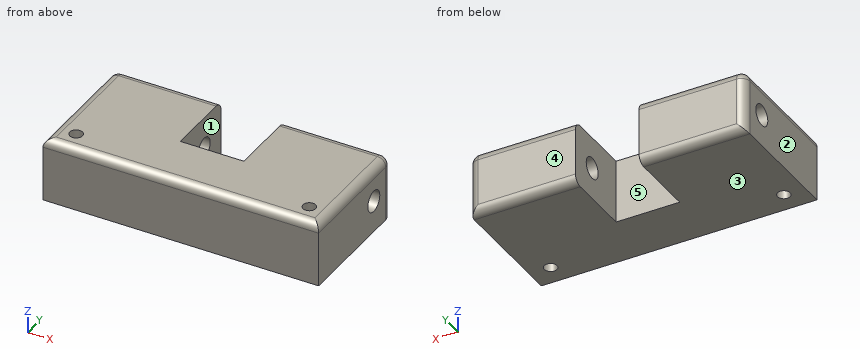
```python
from build123d import *

# Parameters (mm, degrees)
SKETCH1_W           = 65
SKETCH1_H           = 30.1
SKETCH1_R           = 1.5
BOSS_EXTRUDE1_DEPTH = 15
SKETCH2_R           = 2.5
CUT_EXTRUDE1_DEPTH  = 75
SKETCH3_W           = 15
SKETCH3_H           = 17
CUT_EXTRUDE2_DEPTH  = 75
FILLET2_R           = 2


with BuildPart() as part:
    # Sketch1 → Boss-Extrude1 (new body)
    with BuildSketch(Plane.XY):
        with Locations((10, 0.55)):
            Rectangle(SKETCH1_W, SKETCH1_H)
        with Locations((-17.5, -9.5)):
            Circle(SKETCH1_R, mode=Mode.SUBTRACT)
        with Locations((37.5, -9.5)):
            Circle(SKETCH1_R, mode=Mode.SUBTRACT)
    extrude(amount=BOSS_EXTRUDE1_DEPTH)

    # Sketch2 → Cut-Extrude1 (cut)
    with BuildSketch(Plane.ZY.offset(22.5)):
        with Locations((7.5, 8.6)):
            Circle(SKETCH2_R)
    extrude(amount=-CUT_EXTRUDE1_DEPTH, mode=Mode.SUBTRACT)

    # Sketch3 → Cut-Extrude2 (cut)
    with BuildSketch(Plane.XY.offset(15)):
        with Locations((10, 7.1)):
            Rectangle(SKETCH3_W, SKETCH3_H)
    extrude(amount=-CUT_EXTRUDE2_DEPTH, mode=Mode.SUBTRACT)

    # Fillet2
    fillet2_edges = [part.edges().sort_by_distance(p)[0] for p in [
        (42.5, 0.55, 15),
        (30, 15.6, 15),
        (-10, 15.6, 0),
        (-10, 15.6, 15),
        (-22.5, 0.55, 15),
        (30, 15.6, 0),
        (-22.5, 15.6, 7.5),
        (42.5, 15.6, 7.5),
        (10, -14.5, 15),
    ]]
    fillet(fillet2_edges, radius=FILLET2_R)


solid = part.part
```
Can you work these out from the model? Positions are in its coordinate system, mm. Face numbers are marked on the shaded views. A direction names the side the tool comes from. Give positions to 0.01 mm unless a question says otherwise; leave off trailing zeros. Loops run counter-clockwise (first coordinate to the right, second up) from the corner with the lowest first, then second, coordinate; pieces in that order, holes last. Notation, with made-up numbers: M -36,-9.5 L -10,-9.5 A22 cw -10,24.5 Z; hole C 89,-24.75 d10. An arc over 180 degrees is marked long. Use CSV: the item, a comma, the result in double quotes. Start each with the question number.
1. If I drill on L1, parallel to X at y = -0.5, z = 12; L2, parallel to Y at x = 37.5, z = 4; L3, parallel to Y at x = 31.5, z = 7.5, over which ranges is the centre line in solid material (lowest first)?
2. If we mould it in two halves opening along X, with no side actions, what happens to the marked faces 1, 2 and 3? For each: released by +X, released by -X, zero draft, split by the parting line, or undercut.
3. On a 3-axis mill with a long thin cutter (end or side, diameter ignored), from which of +Z, -Z, +X, -X, +Y, -Y can I reach the whole of each face in a straight line? I mean the marked faces 4 and 5. Say none if no direction works.
4. Imagine slicing it at A-A, the plane x = -17.5. Write out the boundary of the cut face in (y, z), plus the area to 3 significant figures.
5. Imagine slicing it at C-C, the plane z = 9. Write out the boundary of the cut face in (x, y), plus the area to 3 significant figures.
6. Imagine slicing it at B-B, the plane y = -9.5. Write out the boundary of the cut face in (x, z).
7. For P1, Ø1.8, axis at x = 37.5, y = -9.5, coming from the +Z side; P2, Ø7.5, axis at x = 6.5, z = 5, coming from the +Y side, each with a flat end and sliding along its axis, tell me the tip position at first contact or that it passes through.
8. Imagine slicing it at D-D, the plane y = 4. Write out the boundary of the cut face in (x, z).
Response values:
1,L1,"-22.5 to 2.5, 17.5 to 42.5"
1,L2,"-14.5 to -11, -8 to 15.6"
1,L3,"-14.5 to 6.1, 11.1 to 15.6"
2,face 1,"undercut"
2,face 2,"released by -X"
2,face 3,"zero draft"
3,face 4,"+Z, -Z, +X, -X, +Y"
3,face 5,"+Z, -Z, +Y"
4,outline,"M -14.5,0 L -11,0 L -11,15 L -12.5,15 A2 ccw -14.5,13 Z; M -8,0 L 13.6,0 A2 ccw 15.6,2 L 15.6,13 A2 ccw 13.6,15 L -8,15 Z; hole C 8.6,7.5 d5"
4,area,"384 mm^2"
5,outline,"M -22.5,-14.5 L 42.5,-14.5 L 42.5,6.6 L 17.5,6.6 L 17.5,-1.4 L 2.5,-1.4 L 2.5,6.6 L -22.5,6.6 Z; M -22.5,10.6 L 2.5,10.6 L 2.5,15.6 L -20.5,15.6 A2 ccw -22.5,13.6 Z; M 17.5,10.6 L 42.5,10.6 L 42.5,13.6 A2 ccw 40.5,15.6 L 17.5,15.6 Z; hole C -17.5,-9.5 d3; hole C 37.5,-9.5 d3"
5,area,"1,490 mm^2"
6,outline,"M -22.5,0 L -19,0 L -19,15 L -20.5,15 A2 ccw -22.5,13 Z; M -16,0 L 36,0 L 36,15 L -16,15 Z; M 39,0 L 42.5,0 L 42.5,13 A2 ccw 40.5,15 L 39,15 Z"
7,P1,"through"
7,P2,"y = -1.4"
8,outline,"M -22.5,0 L 2.5,0 L 2.5,15 L -20.5,15 A2 ccw -22.5,13 Z; M 17.5,0 L 42.5,0 L 42.5,13 A2 ccw 40.5,15 L 17.5,15 Z"
